The figure shows three views and two pictorial views of one solid part (mm, origin at its lowest corner). Answer the questions. Coordinates: 2 decimals unless noted, no trailing zeros. Write each loop counter-clockwise with the first axis right and the second up, starting at its lowest first coordinate (ties: lowest second). Pieces come first, ordered by that corner, then holes.
Item 1: Each of these flat-tipped pins is pushed along its axis until it touches: P1, Ø4, axis at y = 64.5, z = 8.5, coming from the +X side; P2, Ø10, axis at y = 66, z = 11.5, coming from the -X side; P3, Ø5.5, axis at x = 429.5, z = 12, coming from the -Y side; P4, Ø15, axis at x = 457.2, y = 77.47, coming from the -Z side. Where does it stop, or does it pass through?
Item 2: Section B-B (y = 11) is taken. Give the vertices of the cut face in (x, z).
Item 3: Section D-D (y = 77.47) is taken. Give the vertices of the cut face in (x, z), then the cut area to 3 significant figures.
Item 4: Section C-C (z = 3.25) is taken. Give the vertices of the cut face in (x, y), then the cut area to 3 significant figures.
Item 5: Straight lines are drawn through the part: probe 1 along X at (y, z) = (16, 5.5); probe 2 along Y at (x, z) = (152.4, 14.25); probe 3 along X at (y, z) = (61, 5.25). For each, find the intervals that lie inside material, in ascending order.
Item 6: Section A-A (x = 152.4) is taken. Give the vertices of the cut face in (y, z), then the cut area to 3 significant figures.
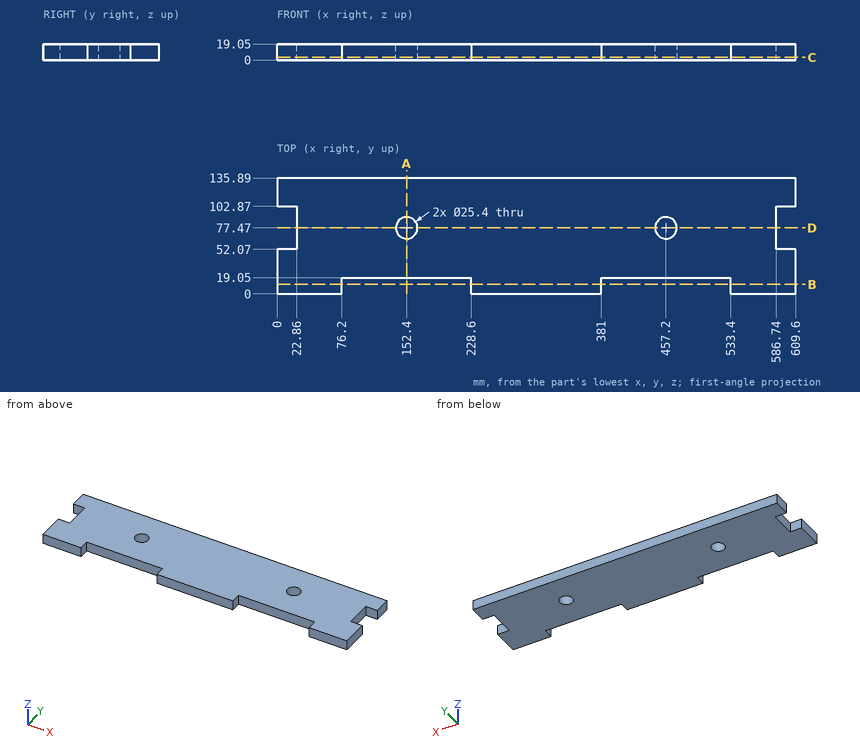
Established:
1. P1: stops at x = 586.74
1. P2: stops at x = 22.86
1. P3: stops at y = 19.05
1. P4: passes through
2. outline: (0, 0) - (76.2, 0) - (76.2, 19.05) - (0, 19.05) - close; (228.6, 0) - (381, 0) - (381, 19.05) - (228.6, 19.05) - close; (533.4, 0) - (609.6, 0) - (609.6, 19.05) - (533.4, 19.05) - close
3. outline: (22.86, 0) - (139.7, 0) - (139.7, 19.05) - (22.86, 19.05) - close; (165.1, 0) - (444.5, 0) - (444.5, 19.05) - (165.1, 19.05) - close; (469.9, 0) - (586.74, 0) - (586.74, 19.05) - (469.9, 19.05) - close
3. area: 9,770 mm2
4. outline: (0, 0) - (76.2, 0) - (76.2, 19.05) - (228.6, 19.05) - (228.6, 0) - (381, 0) - (381, 19.05) - (533.4, 19.05) - (533.4, 0) - (609.6, 0) - (609.6, 52.07) - (586.74, 52.07) - (586.74, 102.87) - (609.6, 102.87) - (609.6, 135.89) - (0, 135.89) - (0, 102.87) - (22.86, 102.87) - (22.86, 52.07) - (0, 52.07) - close; hole circle Ø25.4 at (152.4, 77.47); hole circle Ø25.4 at (457.2, 77.47)
4. area: 73,700 mm2
5. probe 1: x = 0 to 76.2, 228.6 to 381, 533.4 to 609.6
5. probe 2: y = 19.05 to 64.77, 90.17 to 135.89
5. probe 3: x = 22.86 to 586.74
6. outline: (19.05, 0) - (64.77, 0) - (64.77, 19.05) - (19.05, 19.05) - close; (90.17, 0) - (135.89, 0) - (135.89, 19.05) - (90.17, 19.05) - close
6. area: 1,740 mm2
